The drawing under review shows one solid part. Ordinate dimensions are in mm from its lowest x, y, z. A direction names the side the tool comes from. Give positions to 0.01 mm unless a question says otherwise; leave off trailing zeros. Write each loop counter-clockwise with the first axis right and the second up, starting at its lowest first coordinate (ties: lowest second). Pieces come first, ordered by that corner, then holes.
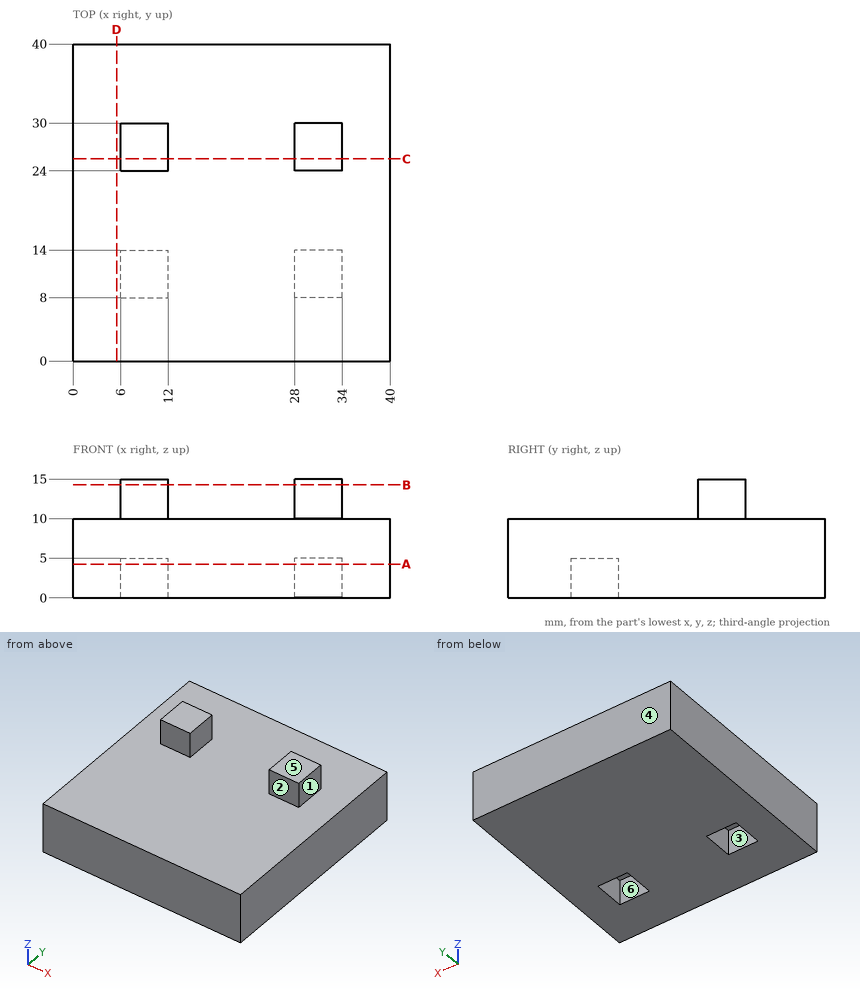
1) The part is to be moulded in two halves that separate along Y. For the marked faces 4, 5 and 6, say which applies: +Y half, -Y half, draft (parallel to the pull), parting line (faces both ways), or undercut.
2) Consider section A-A, the plane z = 4.25. Give the boundary of the cut face in (x, y), then the cut area to 3 significant figures.
3) Consider section D-D, the plane x = 5.5. Give the boundary of the cut face in (y, z), then the cut area to 3 significant figures.
4) Tool access review of the marked faces 1, 2 and 3: name each direction out of +Z, -Z, +X, -X, +Y, -Y from which nothing blocks a thin tool from reaching the whole face with its end or side.
5) Insertion check: pin 1 (1.5 mm diameter, centred on x = 31.5, z = 12, fed in from +Y); pin 2 (12 mm diameter, centred on x = 29.5, y = 15, fed in from +Z); pin 3 (5.5 mm diameter, centred on y = 27, z = 13, fed in from -X). Each pin has a flat end and moves straight along its axis. Give the tip position at first contact, or say it passes through.
6) Consider section B-B, the plane z = 14.25. Give the boundary of the cut face in (x, y).
7) To check wall thickness, follow probe 1 along X at (y, z) = (13, 3.5); probe 2 along Z at (x, y) = (2.5, 30); probe 3 along Y at (x, z) = (32, 14.25). State the ranges of each line that lie inside material, in increasing order.
8) Consider section C-C, the plane y = 25.5. Give the boundary of the cut face in (x, z).
Answer block:
1. face 4: +Y half
1. face 5: draft
1. face 6: undercut
2. outline: (0, 0) - (40, 0) - (40, 40) - (0, 40) - close; hole (6, 8) - (12, 8) - (12, 14) - (6, 14) - close; hole (28, 8) - (34, 8) - (34, 14) - (28, 14) - close
2. area: 1,530 mm2
3. outline: (0, 0) - (40, 0) - (40, 10) - (0, 10) - close
3. area: 400 mm2
4. face 1: +Z, +X, +Y, -Y
4. face 2: +Z, +X, -X, -Y
4. face 3: -Z
5. pin 1: stops at y = 30
5. pin 2: stops at z = 10
5. pin 3: stops at x = 6
6. outline: (6, 24) - (12, 24) - (12, 30) - (6, 30) - close; (28, 24) - (34, 24) - (34, 30) - (28, 30) - close
7. probe 1: x = 0 to 6, 12 to 28, 34 to 40
7. probe 2: z = 0 to 10
7. probe 3: y = 24 to 30
8. outline: (0, 0) - (40, 0) - (40, 10) - (34, 10) - (34, 15) - (28, 15) - (28, 10) - (12, 10) - (12, 15) - (6, 15) - (6, 10) - (0, 10) - close
